```python
from build123d import *

# Parameters (mm, degrees)
BOSS_EXTRUDE1_DEPTH   = 20
BOSS_EXTRUDE1_2_DEPTH = 20
BOSS_EXTRUDE1_3_DEPTH = 20
BOSS_EXTRUDE1_4_DEPTH = 20
SKETCH2_W             = 20
SKETCH2_H             = 20
BOSS_EXTRUDE2_DEPTH   = 20
CUT_EXTRUDE1_DEPTH    = 31


with BuildPart() as part:
    # Sketch1 → Boss-Extrude1 (new body)
    with BuildSketch(Plane(origin=(0, 0, 0), x_dir=(1, 0, 0), z_dir=(0, 1, 0))):
        Polygon((-10, -2.8), (-10, 2.8), (-7.7, 2.8), (-7.7, 5.58), (-7.135634919, 5.58), (-4.28, 2.724365081), (-4.28, -2.724365081), (-7.135634919, -5.58), (-7.7, -5.58), (-7.7, -2.8), align=None)
    extrude(amount=BOSS_EXTRUDE1_DEPTH)



with BuildPart() as body_2:
    # Sketch1 → Boss-Extrude1 2 (new body)
    with BuildSketch(Plane(origin=(0, 0, 0), x_dir=(1, 0, 0), z_dir=(0, 1, 0))):
        Polygon((10, 2.8), (7.7, 2.8), (7.7, 5.58), (7.135634919, 5.58), (4.28, 2.724365081), (4.28, -2.724365081), (7.135634919, -5.58), (7.7, -5.58), (7.7, -2.8), (10, -2.8), align=None)
    extrude(amount=BOSS_EXTRUDE1_2_DEPTH)


with BuildPart() as body_3:
    # Sketch1 → Boss-Extrude1 3 (new body)
    with BuildSketch(Plane(origin=(0, 0, 0), x_dir=(1, 0, 0), z_dir=(0, 1, 0))):
        Polygon((2.8, -10), (-2.8, -10), (-2.8, -7.7), (-5.58, -7.7), (-5.58, -7.135634919), (-2.724365081, -4.28), (2.724365081, -4.28), (5.58, -7.135634919), (5.58, -7.7), (2.8, -7.7), align=None)
    extrude(amount=BOSS_EXTRUDE1_3_DEPTH)


with BuildPart() as body_4:
    # Sketch1 → Boss-Extrude1 4 (new body)
    with BuildSketch(Plane(origin=(0, 0, 0), x_dir=(1, 0, 0), z_dir=(0, 1, 0))):
        Polygon((-2.8, 10), (-2.8, 7.7), (-5.58, 7.7), (-5.58, 7.135634919), (-2.724365081, 4.28), (2.724365081, 4.28), (5.58, 7.135634919), (5.58, 7.7), (2.8, 7.7), (2.8, 10), align=None)
    extrude(amount=BOSS_EXTRUDE1_4_DEPTH)


with BuildPart() as part_1:
    add(part.part)

    add(body_2.part)  # Boss-Extrude2 merges body 2

    add(body_3.part)  # Boss-Extrude2 merges body 3

    add(body_4.part)  # Boss-Extrude2 merges body 4
    # Sketch2 → Boss-Extrude2 (add)
    with BuildSketch(Plane.XZ):
        Rectangle(SKETCH2_W, SKETCH2_H)
    extrude(amount=BOSS_EXTRUDE2_DEPTH)

    # Sketch3 → Cut-Extrude1 (cut, through all)
    with BuildSketch(Plane(origin=(10, 0, 0), x_dir=(0, 0, -1), z_dir=(1, 0, 0))):
        Polygon((10.596673941, -8.137212268), (10.596673941, -38.345549702), (-10.411138478, -38.345549702), (-10.411138478, -2.402671747), align=None)
    extrude(amount=-CUT_EXTRUDE1_DEPTH, mode=Mode.SUBTRACT)


solid = part_1.part
```
The listing builds one solid part. Answer for the finished solid, in the listing's coordinates (mm). A direction names the side the tool comes from. Give positions to 0.01 mm unless a question says otherwise; leave off trailing zeros. Order: outer loops, then holes, each group sorted by start corner. A loop starts at its lowest first (then second) coordinate and runs counter-clockwise, first axis right, second up. Notation, with made-up numbers: (-36.5, -19.75) - (1.5, -19.75) arc R16 cw to (1.5, -6.75) - close; hole circle Ø8 at (45.5, 34.5). An arc over 180 degrees is marked (long way). Answer in a Markdown table with one row per item. Add a question column.
Q1. Given P1, Ø0.7, axis at y = 13, z = -8.5, coming from the -X side; P2, Ø4, axis at y = 7.5, z = -5.5, coming from the +X side; P3, Ø2, axis at x = -4.5, y = 10, coming from the +Z side, each flat-ended and moving along its own axis, determine where each tip first touches the part or whether it passes through.
Q2. The part is cut by section D-D (y = -6). Determine the outline of the cut face in (x, z), then the cut area to 3 significant figures.
Q3. The part is cut by section B-B (z = -3.25). Determine the outline of the cut face in (x, y).
Q4. Which of the six approach directions +Z, -Z, +X, -X, +Y, -Y give full straight-line access (tool end or side, diameter ignored) to faces 1 (the flat face through (-4, 10, 7.7)), 2 (the flat face through (5.728, 9.86, -4.172)), 3 (the flat face through (2.8, 10, -9))?
Q5. Find the intervals of material crossed by line 1 along X through (y, z) = (9.5, -0.5); line 2 along Z through (x, y) = (5.5, 13.5); line 3 along Z through (x, y) = (-4.75, 1.75), in increasing order. Write a range as [from, to].
Q6. The part is cut by section A-A (x = -0.5). Determine the outline of the cut face in (y, z), then the cut area to 3 significant figures.
Q7. For a pull along Z with two mould halves and no side action, classify faces 4 (the flat face through (-4.172, 9.86, -5.728)), 5 (the flat face through (4.132, 9.86, 5.688)), 6 (the flat face through (0.14, -5.206, 0.14)), 7 (the flat face through (-4, 10, -7.7)) as released by +Z, released by -Z, zero draft, split by the parting line, or undercut.
Q8. The part is cut by section C-C (y = 13.25). Give the number of separate pieces and of enclosed holes in the cut face, then the cut area to 3 significant figures.
Determined:
| question | item | result |
|---|---|---|
| 1 | P1 | stops at x = -2.8 |
| 1 | P2 | stops at x = 7.7 |
| 1 | P3 | stops at z = 7.7 |
| 2 | outline | (-10, -10) - (10, -10) - (10, -2.77) - (-10, -2.77) - close |
| 2 | area | 145 mm² |
| 3 | outline | (-10, -6.13) - (10, -6.13) - (10, 0) - (7.7, 0) - (7.7, 20) - (4.81, 20) - (4.81, 0) - (-4.81, 0) - (-4.81, 20) - (-7.7, 20) - (-7.7, 0) - (-10, 0) - close |
| 4 | face 1 | +Z, -X, +Y |
| 4 | face 2 | +Y |
| 4 | face 3 | -Z, +X, +Y |
| 5 | line 1 | x = [-10, -4.28], [4.28, 10] |
| 5 | line 2 | z = [-7.7, -7.06], [-3.94, 3.94], [7.06, 7.7] |
| 5 | line 3 | z = [-7.7, -6.31], [-3.19, 3.19], [6.31, 7.7] |
| 6 | outline | (-7.97, -10) - (20, -10) - (20, -4.28) - (0, -4.28) - (0, 4.28) - (20, 4.28) - (20, 10) - (-2.51, 10) - close |
| 6 | area | 334 mm² |
| 7 | face 4 | undercut |
| 7 | face 5 | undercut |
| 7 | face 6 | released by +Z |
| 7 | face 7 | released by -Z |
| 8 | separate pieces | 4 |
| 8 | enclosed holes | 0 |
| 8 | area | 172 mm² |
